CAD build for the part. Positions are in the model's coordinates, mm. Face numbers are marked on the shaded views. Round coordinates to 2 decimals unless told otherwise and drop trailing zeros. Order: outer loops, then holes, each group sorted by start corner. A loop starts at its lowest first (then second) coordinate and runs counter-clockwise, first axis right, second up. Notation, with made-up numbers: (5.5, 19.25) -> (11.5, 19.25) arc R16 ccw to (11.5, 45.25) -> close; hole circle Ø1 at (59.25, 44.25). An arc over 180 degrees is marked (long way). Return JSON: item names as keys, results as strings. Group by question number.
Q1. Mould opens along Y. For the marked faces 1, 2 and 3 say: +Y half, -Y half, draft (parallel to the pull), parting line (faces both ways), or undercut.
Q2. Cut at A-A (x = 0). Write the cut outline in (y, z).
Q3. Cut at B-B (y = 0). Write the cut outline in (x, z).
Q4. Cut at C-C (z = 2.75). Count the separate pieces of the cut face and the enclosed holes in it, then the cut area to 3 significant figures.
Q5. Flat gauge pins, fed straight in: pin 1 (2.5 mm diameter, centred on x = -11.91, y = 21.43, fed in from -Z); pin 2 (4.5 mm diameter, centred on x = -16.5, y = 9.52, fed in from -Z); pin 3 (4 mm diameter, centred on x = 11.91, y = 21.43, fed in from -Z); pin 4 (5 mm diameter, centred on x = -11.91, y = -21.43, fed in from -Z). Where does each tip first touch, or does it go through?
Q6. Probe line 1 along Y through (x, z) = (-16.5, 5); line 2 along X through (y, z) = (1, 5.75); line 3 along X through (y, z) = (0.5, 4.25). List the from-to ranges inside material, lowest first.
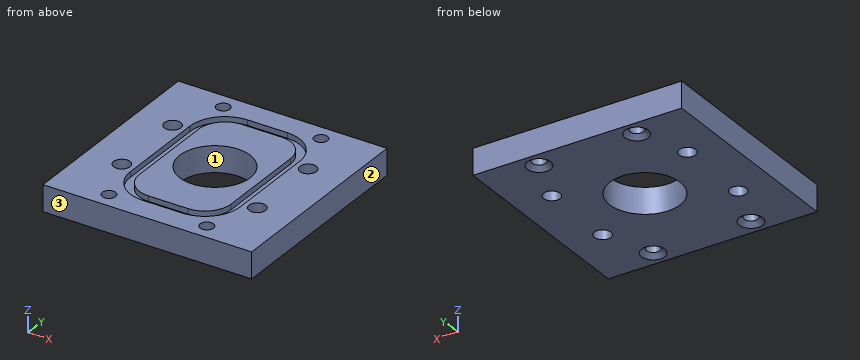
from build123d import *

# Parameters (mm, degrees)
SKETCH1_W                                         = 50.8
SKETCH1_H                                         = 50.8
BOSS_EXTRUDE1_DEPTH                               = 6.35
SKETCH2_R                                         = 8.5852
CUT_EXTRUDE1_DEPTH                                = 7.35
CUT_EXTRUDE2_DASH_027_DEPTH                       = 1.3208
CSK_FOR_4_FLAT_HEAD_MACHINE_SCREW_100_D           = 3.2639
CSK_FOR_4_FLAT_HEAD_MACHINE_SCREW_100_CSINK_D     = 5.715
CSK_FOR_4_FLAT_HEAD_MACHINE_SCREW_100_CSINK_ANGLE = 100
F_10_32_TAPPED_HOLE1_AT_2_COUNT                   = 2
F_10_32_TAPPED_HOLE1_AT_2_PITCH                   = 19.05


with BuildPart() as part:
    # Sketch1 → Boss-Extrude1 (new body)
    with BuildSketch(Plane.XY):
        Rectangle(SKETCH1_W, SKETCH1_H)
    extrude(amount=BOSS_EXTRUDE1_DEPTH)

    # Sketch2 → Cut-Extrude1 (cut, through all)
    with BuildSketch(Plane.XY.offset(6.35)):
        Circle(SKETCH2_R)
    extrude(amount=-CUT_EXTRUDE1_DEPTH, mode=Mode.SUBTRACT)

    # Sketch3 → Cut-Extrude2 - dash 027 (cut)
    with BuildSketch(Plane.XY.offset(6.35)):
        with BuildLine():
            Line((13.3477, -11.176), (13.3477, 11.176))
            ThreePointArc((13.3477, 11.176), (10.848032113, 17.210732113), (4.8133, 19.7104))
            Line((4.8133, 19.7104), (-4.8133, 19.7104))
            ThreePointArc((-4.8133, 19.7104), (-10.848032113, 17.210732113), (-13.3477, 11.176))
            Line((-13.3477, 11.176), (-13.3477, -11.176))
            ThreePointArc((-13.3477, -11.176), (-10.848032113, -17.210732113), (-4.8133, -19.7104))
            Line((-4.8133, -19.7104), (4.8133, -19.7104))
            ThreePointArc((4.8133, -19.7104), (10.848032113, -17.210732113), (13.3477, -11.176))
        make_face()
        with BuildLine():
            Line((-4.8133, -17.526), (4.8133, -17.526))
            ThreePointArc((4.8133, -17.526), (9.303428061, -15.666128061), (11.1633, -11.176))
            Line((11.1633, -11.176), (11.1633, 11.176))
            ThreePointArc((11.1633, 11.176), (9.303428061, 15.666128061), (4.8133, 17.526))
            Line((4.8133, 17.526), (-4.8133, 17.526))
            ThreePointArc((-4.8133, 17.526), (-9.303428061, 15.666128061), (-11.1633, 11.176))
            Line((-11.1633, 11.176), (-11.1633, -11.176))
            ThreePointArc((-11.1633, -11.176), (-9.303428061, -15.666128061), (-4.8133, -17.526))
        make_face(mode=Mode.SUBTRACT)
    extrude(amount=-CUT_EXTRUDE2_DASH_027_DEPTH, mode=Mode.SUBTRACT)

    # CSK for #4 Flat Head Machine Screw (100)1 (through all)
    with Locations(Plane(origin=(0, 0, 0), x_dir=(-1, 0, 0), z_dir=(0, 0, -1))):
        with Locations((-11.90625, 21.43125), (11.90625, 21.43125), (-11.90625, -21.43125), (11.90625, -21.43125)):
            CounterSinkHole(CSK_FOR_4_FLAT_HEAD_MACHINE_SCREW_100_D / 2, CSK_FOR_4_FLAT_HEAD_MACHINE_SCREW_100_CSINK_D / 2, counter_sink_angle=CSK_FOR_4_FLAT_HEAD_MACHINE_SCREW_100_CSINK_ANGLE)

    # Sketch8 → #10-32 Tapped Hole1 (revolve, cut)
    with BuildSketch(Plane(origin=(-16.497783942, 9.525, 0), x_dir=(0, 1, 0), z_dir=(1, 0, 0))):
        Polygon((0, 0), (0, 14.929317848), (2.0193, 13.716), (2.0193, 0), align=None)
    f_10_32_tapped_hole1 = revolve(axis=Axis((-16.497783942, 9.525, -6.35), (0, 0, 1)), mode=Mode.SUBTRACT)

    # #10-32 Tapped Hole1 at 2: #10-32 Tapped Hole1 ×2
    with Locations(*[(0, -i * F_10_32_TAPPED_HOLE1_AT_2_PITCH, 0) for i in range(1, F_10_32_TAPPED_HOLE1_AT_2_COUNT)]):
        add(f_10_32_tapped_hole1, mode=Mode.SUBTRACT)

    # Mirror1: #10-32 Tapped Hole1 across plane
    add(f_10_32_tapped_hole1.mirror(Plane(origin=(0, 0, 0), x_dir=(0, 0, 1), z_dir=(1, 0, 0))), mode=Mode.SUBTRACT)

    # Mirror1 copy 1 sketch → Mirror1 copy 1 (revolve, cut)
    with BuildSketch(Plane(origin=(16.497783942, -9.525, 0), x_dir=(0, 1, 0), z_dir=(-1, 0, 0))):
        Polygon((0, 0), (0, -14.929317848), (2.0193, -13.716), (2.0193, 0), align=None)
    revolve(axis=Axis((16.497783942, -9.525, -6.35), (0, 0, -1)), mode=Mode.SUBTRACT)


solid = part.part
Solution:
{
 "1": {"face 1": "undercut", "face 2": "draft", "face 3": "-Y half"},
 "2": {"outline": "(-25.4, 0) -> (-8.59, 0) -> (-8.59, 6.35) -> (-17.53, 6.35) -> (-17.53, 5.03) -> (-19.71, 5.03) -> (-19.71, 6.35) -> (-25.4, 6.35) -> close; (8.59, 0) -> (25.4, 0) -> (25.4, 6.35) -> (19.71, 6.35) -> (19.71, 5.03) -> (17.53, 5.03) -> (17.53, 6.35) -> (8.59, 6.35) -> close"},
 "3": {"outline": "(-25.4, 0) -> (-8.59, 0) -> (-8.59, 6.35) -> (-11.16, 6.35) -> (-11.16, 5.03) -> (-13.35, 5.03) -> (-13.35, 6.35) -> (-25.4, 6.35) -> close; (8.59, 0) -> (25.4, 0) -> (25.4, 6.35) -> (13.35, 6.35) -> (13.35, 5.03) -> (11.16, 5.03) -> (11.16, 6.35) -> (8.59, 6.35) -> close"},
 "4": {"separate pieces": "1", "enclosed holes": "9", "area": "2,260 mm²"},
 "5": {"pin 1": "passes through", "pin 2": "stops at z = 0", "pin 3": "stops at z = 0.72", "pin 4": "stops at z = 0.3"},
 "6": {"line 1": "y = -25.4 to -11.54, -7.51 to 7.51, 11.54 to 25.4", "line 2": "x = -25.4 to -13.35, -11.16 to -8.53, 8.53 to 11.16, 13.35 to 25.4", "line 3": "x = -25.4 to -8.57, 8.57 to 25.4"}
}
